Check sheet for the drawn part. Datum: minimum x, y, z corner. Units: mm. Round coordinates to 2 decimals unless told otherwise and drop trailing zeros. Write each loop counter-clockwise with the first axis right and the second up, starting at its lowest first coordinate (ties: lowest second). Pieces come first, ordered by that corner, then holes.
Item 1: Cross-section at C-C on x = 15.4. Enter the section's corners in (y, z).
Item 2: Cross-section at A-A on y = 2.5. Count the separate pieces of the cut face and the enclosed holes in it.
Item 3: Material ranges on line 1 (X direction, y = 1.75, z = 13.5); line 2 (Z direction, x = 22.5, y = 3.2); line 3 (X direction, y = 4.45, z = 13.5), recorded low to high.
Item 4: Cross-section at D-D on x = 37.5. Enter the section's corners in (y, z).
Item 5: Go/stop test with flat-tipped pins: pin 1 Ø5.5 at (x, z) = (22.5, 6.4) entering from -Y; pin 2 Ø5 at (x, z) = (8, 23.5) entering from -Y; pin 3 Ø3 at (x, y) = (37.5, 2) entering from +Z; pin 4 Ø0.6 at (x, y) = (39.5, 3) entering from +Z. Record where each tip stops, or that it passes through.
Item 6: Release check for a two-part mould opening along X. For the marked faces 1, 2, 3 and 4 record: +X half, -X half, draft (parallel to the pull), parting line (faces both ways), or undercut.
Item 7: Cross-section at B-B on z = 22. Enter the section's corners in (x, y).
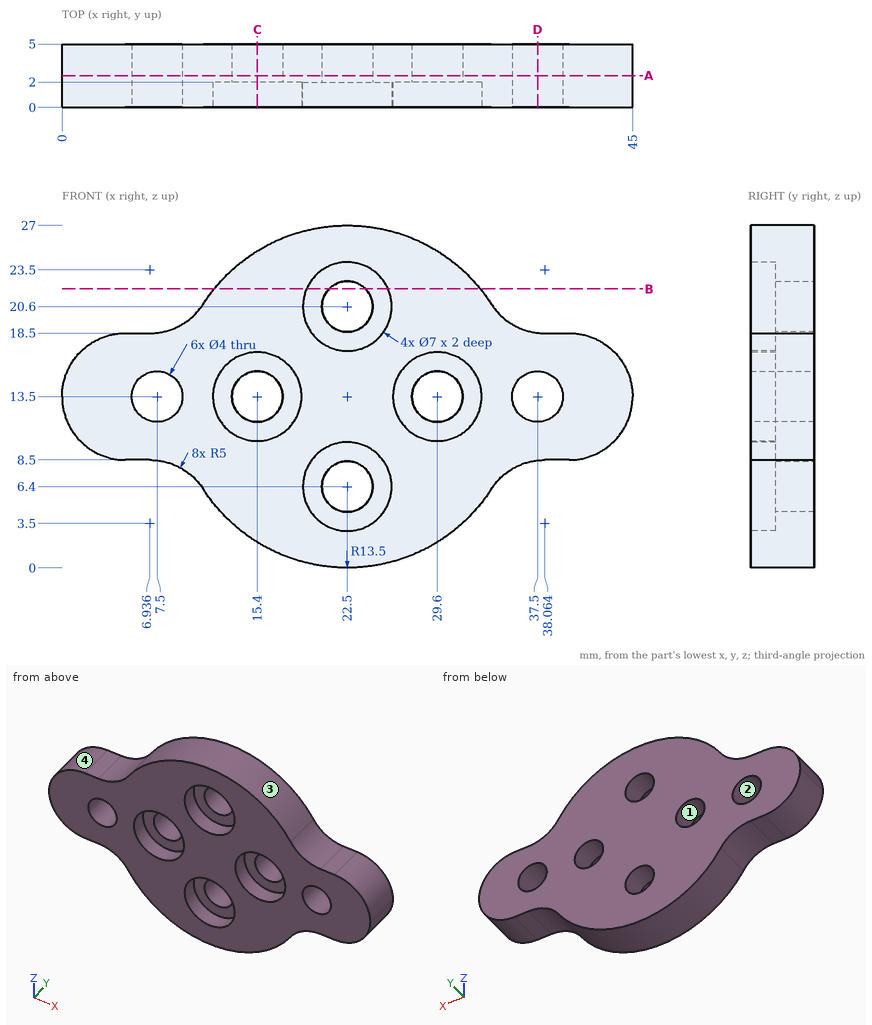
Response values:
1. outline: (0, 2.02) - (5, 2.02) - (5, 11.5) - (2, 11.5) - (2, 10) - (0, 10) - close; (0, 17) - (2, 17) - (2, 15.5) - (5, 15.5) - (5, 24.98) - (0, 24.98) - close
2. separate pieces: 1
2. enclosed holes: 6
3. line 1: x = 0 to 5.5, 9.5 to 11.9, 18.9 to 26.1, 33.1 to 35.5, 39.5 to 45
3. line 2: z = 0 to 4.4, 8.4 to 18.6, 22.6 to 27
3. line 3: x = 0 to 5.5, 9.5 to 13.4, 17.4 to 27.6, 31.6 to 35.5, 39.5 to 45
4. outline: (0, 8.47) - (5, 8.47) - (5, 11.5) - (0, 11.5) - close; (0, 15.5) - (5, 15.5) - (5, 18.53) - (0, 18.53) - close
5. pin 1: stops at y = 2
5. pin 2: passes through
5. pin 3: stops at z = 18.95
5. pin 4: stops at z = 18.5
6. face 1: undercut
6. face 2: undercut
6. face 3: parting line
6. face 4: -X half
7. outline: (12.01, 0) - (19.29, 0) - (19.29, 2) - (21.07, 2) - (21.07, 5) - (12.01, 5) - close; (23.93, 2) - (25.71, 2) - (25.71, 0) - (32.99, 0) - (32.99, 5) - (23.93, 5) - close
